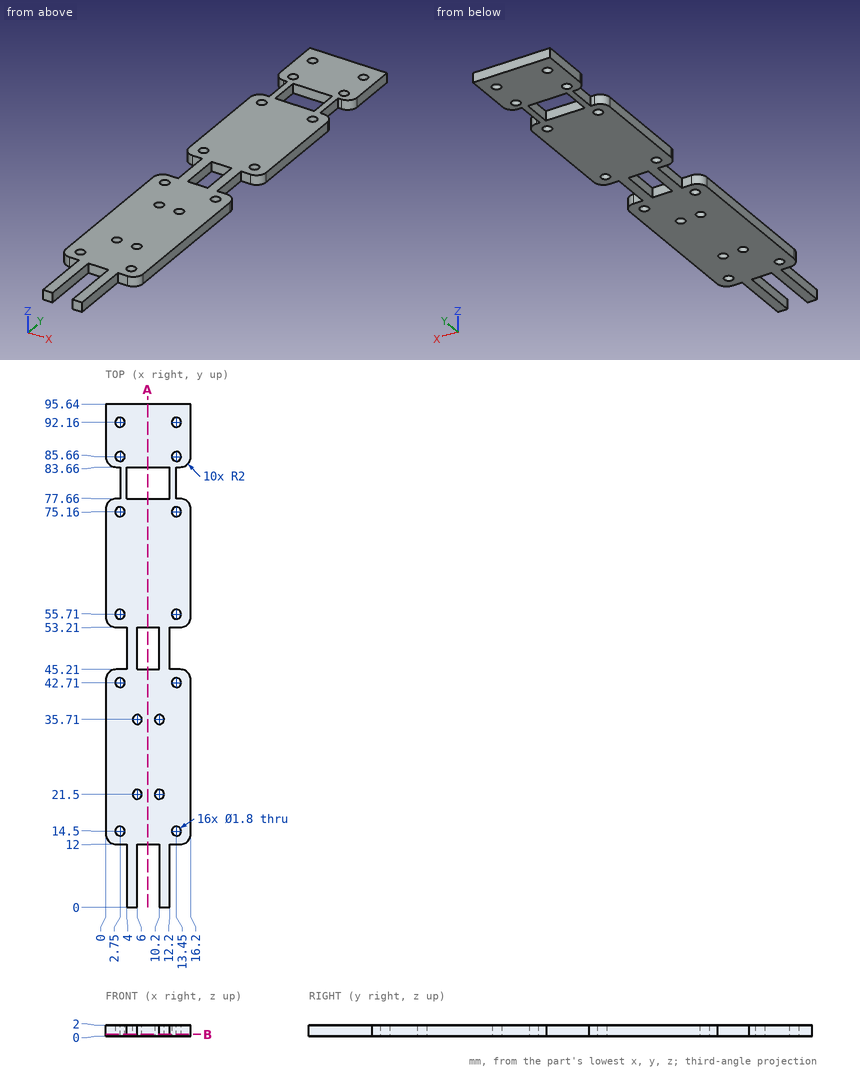
Design review of the part shown in the three views and the two pictorial views. Dimensions are in mm from the part's minimum x, y and z. Give positions to 0.01 mm unless a question says otherwise; leave off trailing zeros. Write each loop counter-clockwise with the first axis right and the second up, starting at its lowest first coordinate (ties: lowest second). Pieces come first, ordered by that corner, then holes. Notation, with made-up numbers: M -24,-34.75 L 6,-34.75 A10 ccw 6,-23.75 Z; hole C -12.75,64 d4. An arc over 180 degrees is marked long. One line per item, written item: value.
1) Take a section at B-B, the plane z = 0.3. Count the separate pieces of the cut face and the enclosed holes in it, then the cut area to 3 significant figures.
Results are:
separate pieces: 1
enclosed holes: 18
area: 1,170 mm²
2) For line 1 (X direction, y = 92.16, z = 1.25); line 2 (Y direction, x = 8.5, z = 1.65); line 3 (Y direction, x = 11.5, z = 1.05), list the stretches that pass through material, from the lowest coordinate up. Write a range as from..to.
Results are:
line 1: x = 0..1.85, 3.65..12.55, 14.35..16.2
line 2: y = 12..45.21, 53.21..77.66, 83.66..95.64
line 3: y = 0..77.66, 83.66..95.64
3) For P1, Ø0.6, axis at x = 13.5, z = 1, coming from the -Y side; P2, Ø2, axis at x = 2.75, y = 42.71, coming from the +Z side; P3, Ø1.6, axis at x = 13.45, y = 42.71, coming from the -Z side; P4, Ø1, axis at y = 50, z = 0.5, coming from the -X side, all flat-tipped, find the tip position at first contact; note any pin that passes through.
Results are:
P1: stops at y = 12
P2: stops at z = 2
P3: passes through
P4: stops at x = 4
4) Take a section at A-A, the plane x = 8. Write out the cut boundary in (y, z), then the cut area to 3 significant figures.
Results are:
outline: M 12,0 L 45.21,0 L 45.21,2 L 12,2 Z; M 53.21,0 L 77.66,0 L 77.66,2 L 53.21,2 Z; M 83.66,0 L 95.64,0 L 95.64,2 L 83.66,2 Z
area: 139 mm²
